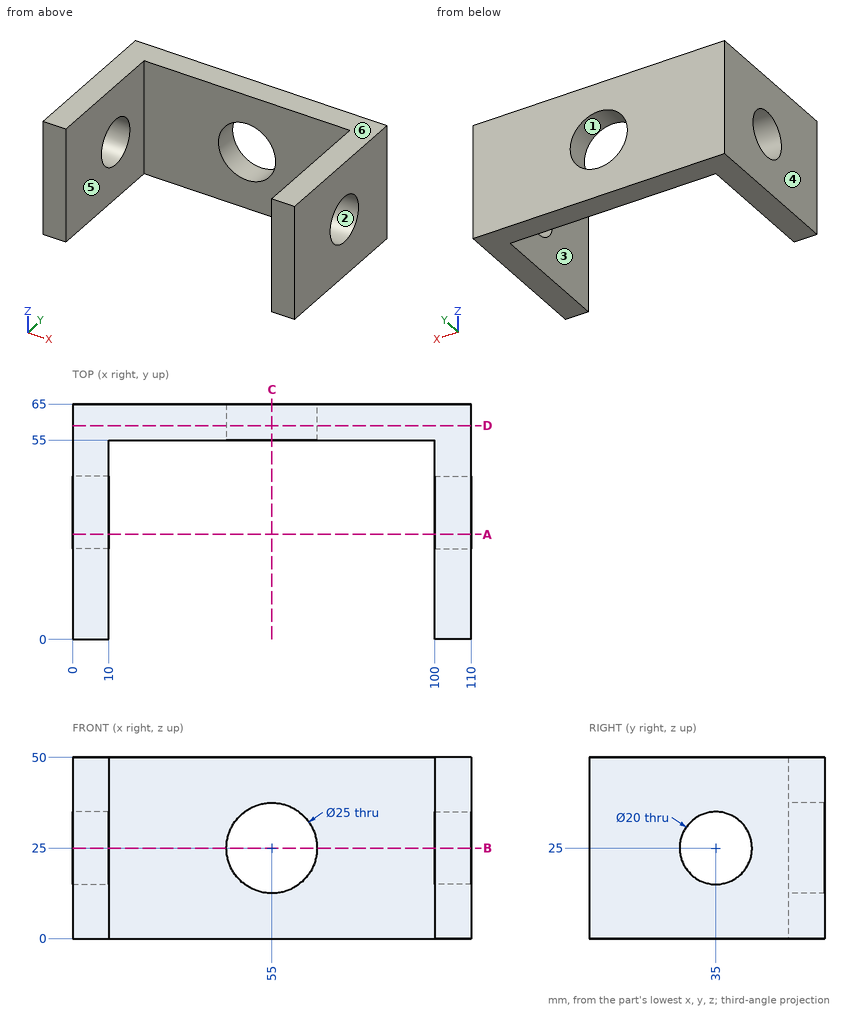
The drawing under review shows one solid part. Ordinate dimensions are in mm from its lowest x, y, z. A direction names the side the tool comes from. Coordinates: 2 decimals unless noted, no trailing zeros. Write each loop counter-clockwise with the first axis right and the second up, starting at its lowest first coordinate (ties: lowest second). Pieces come first, ordered by that corner, then holes.
1) Add section C-C (x = 55). Write out the cut boundary in (y, z), plus the area to 3 significant figures.
2) To check wall thickness, follow L1, parallel to X at y = 50.5, z = 47; L2, parallel to X at y = 62, z = 25; L3, parallel to Z at x = 55, y = 60.75. State the ranges of each line that lie inside material, in increasing order.
3) Add section A-A (y = 29). Write out the cut boundary in (x, z).
4) Mouldability with a two-part tool opening along X and no side actions: class the marked faces 1, 2, 3 and 4 as +X half, -X half, draft (parallel to the pull), parting line (faces both ways), or undercut.
5) Add section D-D (y = 59). Write out the cut boundary in (x, z), plus the area to 3 significant figures.
6) Machinability: for the marked faces 5 and 6, which of the approach directions +Z, -Z, +X, -X, +Y, -Y give a long, thin tool a straight path to every point of the face, cutting with its end or side? Answer none if there is none.
7) Add section B-B (z = 25). Write out the cut boundary in (x, y), plus the area to 3 significant figures.
8) Insertion check: pin 1 (10 mm diameter, centred on x = 69, y = 51.5, fed in from -Z); pin 2 (6 mm diameter, centred on x = 25, z = 36, fed in from -Y). Each pin has a flat end and moves straight along its axis. Give the tip position at first contact, or say it passes through.
Check result:
1. outline: (55, 0) - (65, 0) - (65, 12.5) - (55, 12.5) - close; (55, 37.5) - (65, 37.5) - (65, 50) - (55, 50) - close
1. area: 250 mm2
2. L1: x = 0 to 10, 100 to 110
2. L2: x = 0 to 42.5, 67.5 to 110
2. L3: z = 0 to 12.5, 37.5 to 50
3. outline: (0, 0) - (10, 0) - (10, 17) - (0, 17) - close; (0, 33) - (10, 33) - (10, 50) - (0, 50) - close; (100, 0) - (110, 0) - (110, 17) - (100, 17) - close; (100, 33) - (110, 33) - (110, 50) - (100, 50) - close
4. face 1: undercut
4. face 2: draft
4. face 3: undercut
4. face 4: -X half
5. outline: (0, 0) - (110, 0) - (110, 50) - (0, 50) - close; hole circle Ø25 at (55, 25)
5. area: 5,010 mm2
6. face 5: +Z, -Z, -Y
6. face 6: +Z, +X, -X, +Y, -Y
7. outline: (0, 0) - (10, 0) - (10, 25) - (0, 25) - close; (0, 45) - (10, 45) - (10, 55) - (42.5, 55) - (42.5, 65) - (0, 65) - close; (67.5, 55) - (100, 55) - (100, 45) - (110, 45) - (110, 65) - (67.5, 65) - close; (100, 0) - (110, 0) - (110, 25) - (100, 25) - close
7. area: 1,550 mm2
8. pin 1: stops at z = 0
8. pin 2: stops at y = 55
